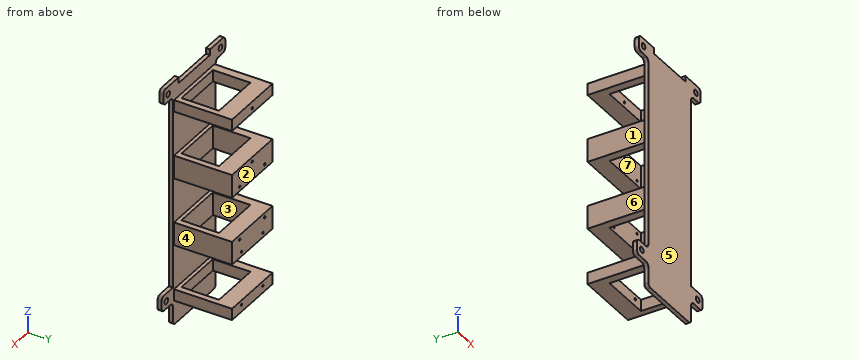
from build123d import *

# Parameters (mm, degrees)
BOSS_EXTRUDE1_DEPTH      = 2.09999993
SKETCH2_R                = 1.5
CUT_EXTRUDE1_DEPTH       = 70.736597565
SKETCH3_R                = 1.5
CUT_EXTRUDE2_DEPTH       = 70.736597565
SKETCH4_R                = 1.5
CUT_EXTRUDE3_DEPTH       = 70.736597565
SKETCH5_R                = 1.5
CUT_EXTRUDE4_DEPTH       = 70.736597565
SKETCH7_W                = 34
SKETCH7_H                = 6
BOSS_EXTRUDE2_DEPTH      = 30
SKETCH8_W                = 34
SKETCH8_H                = 12
BOSS_EXTRUDE3_DEPTH      = 30
SKETCH9_W                = 34
SKETCH9_H                = 12
BOSS_EXTRUDE4_DEPTH      = 30
SKETCH10_W               = 34
SKETCH10_H               = 6
BOSS_EXTRUDE5_DEPTH      = 30
SKETCH11_R               = 0.6
CUT_EXTRUDE5_DEPTH       = 10
SKETCH12_R               = 0.6
CUT_EXTRUDE6_DEPTH       = 10
SKETCH14_R               = 0.6
CUT_EXTRUDE7_DEPTH       = 10
SKETCH13_R               = 0.6
CUT_EXTRUDE8_DEPTH       = 10
SKETCH16_R               = 0.6
CUT_EXTRUDE9_DEPTH       = 10
SKETCH15_R               = 0.6
CUT_EXTRUDE10_DEPTH      = 10
SKETCH17_R               = 0.6
CUT_EXTRUDE11_DEPTH      = 10
SKETCH18_R               = 0.6
CUT_EXTRUDE12_DEPTH      = 10
SKETCH20_R               = 0.6
CUT_EXTRUDE13_DEPTH      = 10
SKETCH19_R               = 0.6
CUT_EXTRUDE14_DEPTH      = 10
CUT_EXTRUDE15_DEPTH      = 126.548171577
CUT_EXTRUDE15_DEPTH_BACK = 126.548171577
SKETCH22_W               = 26.418699501
SKETCH22_H               = 19.436632357


with BuildPart() as part:
    # Sketch1 → Boss-Extrude1 (new body)
    with BuildSketch(Plane(origin=(0, 0, 0), x_dir=(1, 0, 0), z_dir=(0, 1, 0))):
        Polygon((25.50129313, 44.066425413), (18.00129097, 44.066425413), (18.00129097, -54.056063294), (18.069439568, -54.573696107), (18.269239925, -55.056061596), (18.587077968, -55.470272899), (19.001291133, -55.788110942), (19.483652897, -55.987913162), (20.001291297, -56.056059897), (24.001291953, -56.056059897), (24.517572485, -56.123651564), (24.999051355, -56.321874261), (25.413271971, -56.637369096), (25.73231142, -57.048864663), (25.934667327, -57.528622448), (26.006695814, -58.044299483), (26.006695814, -62.047317624), (25.937941857, -62.565967441), (25.737368502, -63.049182296), (25.418632664, -63.464075327), (25.003428571, -63.782408834), (24.52001255, -63.982509077), (24.001291953, -64.050756395), (13.197834603, -64.050756395), (13.197834603, -61.034627259), (-13.188291341, -61.034627259), (-13.188291341, -64.049042761), (-23.998708464, -64.049042761), (-24.518161081, -63.978843391), (-25.001873262, -63.776887953), (-25.417032652, -63.456892967), (-25.735481642, -63.040532172), (-25.935621001, -62.55607307), (-26.003879495, -62.03635782), (-26.003879495, -58.053664863), (-25.953554548, -57.608105242), (-25.805114768, -57.18498677), (-25.566042401, -56.805640459), (-25.248377584, -56.489177048), (-24.868131615, -56.25154078), (-24.444459938, -56.104697287), (-23.998708464, -56.056059897), (-19.996122457, -56.056059897), (-19.478482194, -55.987913162), (-18.996122293, -55.788110942), (-18.581907265, -55.470272899), (-18.264069222, -55.056061596), (-18.064268865, -54.573696107), (-17.996122129, -54.056063294), (-17.996122129, 42.067930102), (-18.064268865, 42.585570365), (-18.264069222, 43.067932129), (-18.581907265, 43.482143432), (-18.996122293, 43.799981475), (-19.478482194, 43.999779969), (-19.996122457, 44.06793043), (-25.498564355, 44.06793043), (-26.016111486, 44.136047363), (-26.498408057, 44.335756451), (-26.912606321, 44.653456658), (-27.230496518, 45.067507774), (-27.430427261, 45.549713075), (-27.498778887, 46.067230403), (-27.50061173, 50.064973533), (-27.450750582, 50.510723144), (-27.302895673, 50.934184343), (-27.064475231, 51.314093173), (-26.747453026, 51.631387323), (-26.367745362, 51.870137453), (-25.944414549, 52.018359303), (-25.498707779, 52.068602294), (-19.996122457, 52.068602294), (-19.478482194, 52.136752754), (-18.996122293, 52.336554974), (-18.581907265, 52.654393017), (-18.264069222, 53.06860432), (-18.064268865, 53.550966084), (-17.996122129, 54.068602622), (-17.996122129, 62.050756067), (-17.927971669, 62.56839633), (-17.728171311, 63.050758094), (-17.410335131, 63.464969397), (-16.996121965, 63.782811165), (-16.513758339, 63.982609659), (-15.996121801, 64.050756395), (16.001292504, 64.050756395), (16.518929042, 63.982609659), (17.001292668, 63.782811165), (17.415505834, 63.464969397), (17.733342014, 63.050758094), (17.933142371, 62.56839633), (18.00129097, 62.050756067), (18.00129097, 54.065614939), (18.069439568, 53.547978401), (18.269239925, 53.065616637), (18.587077968, 52.651405334), (19.001291133, 52.333563566), (19.483652897, 52.133765072), (20.001291297, 52.065614611), (25.504794903, 52.065614611), (26.021647267, 51.996443421), (26.503062807, 51.796041429), (26.916333474, 51.478035748), (27.233376168, 51.064021885), (27.432647534, 50.582136959), (27.50061173, 50.065122545), (27.50061173, 46.100758016), (27.457182296, 45.650146902), (27.313507162, 45.220848173), (27.076949365, 44.834870845), (26.759632863, 44.511999935), (26.377822272, 44.268775731), (25.951082818, 44.117670506), align=None)
    extrude(amount=BOSS_EXTRUDE1_DEPTH)

    # Sketch2 → Cut-Extrude1 (cut, through all)
    with BuildSketch(Plane(origin=(0, 2.09999993, 0), x_dir=(1, 0, 0), z_dir=(0, 1, 0))):
        with Locations(Location((-21.998708135, -60.049042761, 0), (0, 0, 270))):
            Circle(SKETCH2_R)
    extrude(amount=-CUT_EXTRUDE1_DEPTH, mode=Mode.SUBTRACT)

    # Sketch3 → Cut-Extrude2 (cut, through all)
    with BuildSketch(Plane(origin=(0, 2.09999993, 0), x_dir=(1, 0, 0), z_dir=(0, 1, 0))):
        with Locations(Location((22.006695814, -60.056059897, 0), (0, 0, 270))):
            Circle(SKETCH3_R)
    extrude(amount=-CUT_EXTRUDE2_DEPTH, mode=Mode.SUBTRACT)

    # Sketch4 → Cut-Extrude3 (cut, through all)
    with BuildSketch(Plane(origin=(0, 2.09999993, 0), x_dir=(1, 0, 0), z_dir=(0, 1, 0))):
        with Locations(Location((-23.499696034, 48.068602294, 0), (0, 0, 270))):
            Circle(SKETCH4_R)
    extrude(amount=-CUT_EXTRUDE3_DEPTH, mode=Mode.SUBTRACT)

    # Sketch5 → Cut-Extrude4 (cut, through all)
    with BuildSketch(Plane(origin=(0, 2.09999993, 0), x_dir=(1, 0, 0), z_dir=(0, 1, 0))):
        with Locations(Location((23.50061173, 48.066425413, 0), (0, 0, 270))):
            Circle(SKETCH5_R)
    extrude(amount=-CUT_EXTRUDE4_DEPTH, mode=Mode.SUBTRACT)

    # Sketch7 → Boss-Extrude2 (add)
    with BuildSketch(Plane(origin=(0, 2.09999993, 0), x_dir=(1, 0, 0), z_dir=(0, 1, 0))):
        with Locations((0.04381812, 48.432104122)):
            Rectangle(SKETCH7_W, SKETCH7_H)
    extrude(amount=BOSS_EXTRUDE2_DEPTH)

    # Sketch8 → Boss-Extrude3 (add)
    with BuildSketch(Plane(origin=(0, 2.09999993, 0), x_dir=(1, 0, 0), z_dir=(0, 1, 0))):
        with Locations((0.04381812, 16.232104122)):
            Rectangle(SKETCH8_W, SKETCH8_H)
    extrude(amount=BOSS_EXTRUDE3_DEPTH)

    # Sketch9 → Boss-Extrude4 (add)
    with BuildSketch(Plane(origin=(0, 2.09999993, 0), x_dir=(1, 0, 0), z_dir=(0, 1, 0))):
        with Locations((0.04381812, -18.967895878)):
            Rectangle(SKETCH9_W, SKETCH9_H)
    extrude(amount=BOSS_EXTRUDE4_DEPTH)

    # Sketch10 → Boss-Extrude5 (add)
    with BuildSketch(Plane(origin=(0, 2.09999993, 0), x_dir=(1, 0, 0), z_dir=(0, 1, 0))):
        with Locations((0.04381812, -51.167895878)):
            Rectangle(SKETCH10_W, SKETCH10_H)
    extrude(amount=BOSS_EXTRUDE5_DEPTH)

    # Sketch11 → Cut-Extrude5 (cut)
    with BuildSketch(Plane(origin=(0, 32.09999993, 0), x_dir=(1, 0, 0), z_dir=(0, 1, 0))):
        with Locations(Location((-8.95618188, 47.782104122, 0), (0, 0, 270))):
            Circle(SKETCH11_R)
    extrude(amount=-CUT_EXTRUDE5_DEPTH, mode=Mode.SUBTRACT)

    # Sketch12 → Cut-Extrude6 (cut)
    with BuildSketch(Plane(origin=(0, 32.09999993, 0), x_dir=(1, 0, 0), z_dir=(0, 1, 0))):
        with Locations(Location((9.04381812, 47.782104122, 0), (0, 0, 270))):
            Circle(SKETCH12_R)
    extrude(amount=-CUT_EXTRUDE6_DEPTH, mode=Mode.SUBTRACT)

    # Sketch14 → Cut-Extrude7 (cut)
    with BuildSketch(Plane(origin=(0, 32.09999993, 0), x_dir=(1, 0, 0), z_dir=(0, 1, 0))):
        with Locations(Location((9.04381812, 19.882104122, 0), (0, 0, 270))):
            Circle(SKETCH14_R)
    extrude(amount=-CUT_EXTRUDE7_DEPTH, mode=Mode.SUBTRACT)

    # Sketch13 → Cut-Extrude8 (cut)
    with BuildSketch(Plane(origin=(0, 32.09999993, 0), x_dir=(1, 0, 0), z_dir=(0, 1, 0))):
        with Locations(Location((-8.95618188, 19.882104122, 0), (0, 0, 270))):
            Circle(SKETCH13_R)
    extrude(amount=-CUT_EXTRUDE8_DEPTH, mode=Mode.SUBTRACT)

    # Sketch16 → Cut-Extrude9 (cut)
    with BuildSketch(Plane(origin=(0, 32.09999993, 0), x_dir=(1, 0, 0), z_dir=(0, 1, 0))):
        with Locations(Location((10.54381812, 12.582104122, 0), (0, 0, 270))):
            Circle(SKETCH16_R)
    extrude(amount=-CUT_EXTRUDE9_DEPTH, mode=Mode.SUBTRACT)

    # Sketch15 → Cut-Extrude10 (cut)
    with BuildSketch(Plane(origin=(0, 32.09999993, 0), x_dir=(1, 0, 0), z_dir=(0, 1, 0))):
        with Locations(Location((-10.45618188, 12.582104122, 0), (0, 0, 270))):
            Circle(SKETCH15_R)
    extrude(amount=-CUT_EXTRUDE10_DEPTH, mode=Mode.SUBTRACT)

    # Sketch17 → Cut-Extrude11 (cut)
    with BuildSketch(Plane(origin=(0, 32.09999993, 0), x_dir=(1, 0, 0), z_dir=(0, 1, 0))):
        with Locations(Location((-10.45618188, -15.317895878, 0), (0, 0, 270))):
            Circle(SKETCH17_R)
    extrude(amount=-CUT_EXTRUDE11_DEPTH, mode=Mode.SUBTRACT)

    # Sketch18 → Cut-Extrude12 (cut)
    with BuildSketch(Plane(origin=(0, 32.09999993, 0), x_dir=(1, 0, 0), z_dir=(0, 1, 0))):
        with Locations(Location((10.54381812, -15.317895878, 0), (0, 0, 270))):
            Circle(SKETCH18_R)
    extrude(amount=-CUT_EXTRUDE12_DEPTH, mode=Mode.SUBTRACT)

    # Sketch20 → Cut-Extrude13 (cut)
    with BuildSketch(Plane(origin=(0, 32.09999993, 0), x_dir=(1, 0, 0), z_dir=(0, 1, 0))):
        with Locations(Location((0, -50.767895878, 0), (0, 0, 270))):
            Circle(SKETCH20_R)
    extrude(amount=-CUT_EXTRUDE13_DEPTH, mode=Mode.SUBTRACT)

    # Sketch19 → Cut-Extrude14 (cut)
    with BuildSketch(Plane(origin=(0, 32.09999993, 0), x_dir=(1, 0, 0), z_dir=(0, 1, 0))):
        with Locations(Location((0, -22.617895878, 0), (0, 0, 270))):
            Circle(SKETCH19_R)
    extrude(amount=-CUT_EXTRUDE14_DEPTH, mode=Mode.SUBTRACT)

    # Sketch22 → Cut-Extrude15 (cut, two sides: drawn at the far end of the back side and taken through both)
    with BuildSketch(Plane.XY.offset(54.167895878).offset(-CUT_EXTRUDE15_DEPTH_BACK)):
        with Locations((0.682172991, 13.711555244)):
            Rectangle(SKETCH22_W, SKETCH22_H)
    extrude(amount=CUT_EXTRUDE15_DEPTH + CUT_EXTRUDE15_DEPTH_BACK, mode=Mode.SUBTRACT)


solid = part.part
For this review, take the finished solid that the model builds, in its own axes (mm). Face numbers are marked on the shaded views. A direction names the side the tool comes from. Round coordinates to 2 decimals unless told otherwise and drop trailing zeros. Order: outer loops, then holes, each group sorted by start corner. A loop starts at its lowest first (then second) coordinate and runs counter-clockwise, first axis right, second up. Notation, with made-up numbers: M 86,71.25 L 134,71.25 A20 cw 134,107.25 Z; hole C 38.25,85 d1. An arc over 180 degrees is marked long. Use a Markdown table: item, result. Add a question column.
Item 1: Add section A-A, the plane y = 26.5. State how many separate pieces and enclosed holes the cut face has, then the cut area to 3 significant figures.
Item 2: To check wall thickness, follow line 1 along Z through (x, y) = (15, 30); line 2 along Z through (x, y) = (9, 30); line 3 along X through (y, z) = (6, 19). State the ranges of each line that lie inside material, in increasing order.
Item 3: Tool access review of the marked faces 1, 2, 3 and 4: name each direction out of +Z, -Z, +X, -X, +Y, -Y from which nothing blocks a thin tool from reaching the whole face with its end or side.
Item 4: Insertion check: pin 1 (2.5 mm diameter, centred on y = 1.5, z = 62.5, fed in from +X); pin 2 (9.5 mm diameter, centred on y = 13, z = -15, fed in from +X); pin 3 (10 mm diameter, centred on x = 14.5, z = -27.5, fed in from +Y). Each pin has a flat end and moves straight along its axis. Give the tip position at first contact, or say it passes through.
Item 5: Mouldability with a two-part tool opening along X and no side actions: class the marked faces 5, 6 and 7 as released by +X, released by -X, zero draft, split by the parting line, or undercut.
Item 6: Add section C-C, the plane z = 31.5. Give the boundary of the cut face in (x, y), then the cut area to 3 significant figures.
Geometry results:
| question | item | result |
|---|---|---|
| 1 | separate pieces | 4 |
| 1 | enclosed holes | 10 |
| 1 | area | 1,210 mm² |
| 2 | line 1 | z = -51.43 to -45.43, -22.23 to -10.23, 12.97 to 24.97, 48.17 to 54.17 |
| 2 | line 2 | z = -51.43 to -48.38, -47.18 to -45.43, -22.23 to -20.48, -19.28 to -10.23, 12.97 to 24.97, 48.17 to 54.17 |
| 2 | line 3 | x = -16.96 to -12.53, 13.89 to 17.04 |
| 3 | face 1 | +Z, -Z, -X, +Y |
| 3 | face 2 | +Z, -Z, +X, -X, +Y |
| 3 | face 3 | +Z, -Z |
| 3 | face 4 | +Z, -Z, +X, +Y |
| 4 | pin 1 | stops at x = 26.01 |
| 4 | pin 2 | stops at x = 17.04 |
| 4 | pin 3 | stops at y = 2.1 |
| 5 | face 5 | zero draft |
| 5 | face 6 | released by -X |
| 5 | face 7 | undercut |
| 6 | outline | M -18,0 L 18,0 L 18,2.1 L -18,2.1 Z |
| 6 | area | 75.6 mm² |
